```python
from build123d import *

# Parameters (mm, degrees)
SKETCH_2_R      = 2.5
EXTRUDE_1_DEPTH = 5
SKETCH_3_R      = 10
EXTRUDE_2_DEPTH = 1
EXTRUDE_3_DEPTH = 3
CHAMFER_1_SIZE  = 0.5


with BuildPart() as part:
    # 草图2 → 凸台-拉伸1 (new body)
    with BuildSketch(Plane(origin=(0, 0, 0), x_dir=(1, 0, 0), z_dir=(0, 1, 0))):
        with Locations(Location((0, 0, 0), (0, 0, 270))):
            Circle(SKETCH_2_R)
    extrude(amount=EXTRUDE_1_DEPTH)

    # 草图3 → 凸台-拉伸2 (add)
    with BuildSketch(Plane(origin=(0, 5, 0), x_dir=(1, 0, 0), z_dir=(0, 1, 0))):
        with Locations(Location((0, 0, 0), (0, 0, 270))):
            Circle(SKETCH_3_R)
    extrude(amount=EXTRUDE_2_DEPTH)

    # 草图4 → 凸台-拉伸3 (add)
    with BuildSketch(Plane(origin=(0, 6, 0), x_dir=(1, 0, 0), z_dir=(0, 1, 0))):
        Polygon((3.464101615, 6), (-3.464101615, 6), (-6.92820323, 0), (-3.464101615, -6), (3.464101615, -6), (6.92820323, 0), align=None)
    extrude(amount=EXTRUDE_3_DEPTH)

    # 草图8 → 切除-旋转1 (revolve, cut)
    with BuildSketch(Plane.XY, mode=Mode.PRIVATE) as cut_revolve_1_sk:
        Polygon((-6.92820323, 9), (-5.92820323, 9), (-6.92820323, 8.422649731), align=None)
    revolve(cut_revolve_1_sk.sketch.rotate(Axis((0, 0, 0), (0, 1, 0)), 270), axis=Axis((0, 0, 0), (0, 1, 0)), mode=Mode.SUBTRACT)

    # 倒角1
    chamfer_1_edges = [part.edges().sort_by_distance(p)[0] for p in [
        (0, 0, -2.5),
    ]]
    chamfer(chamfer_1_edges, length=CHAMFER_1_SIZE)


solid = part.part
```
CAD build for the part. Positions are in the model's coordinates, mm. A direction names the side the tool comes from. Round coordinates to 2 decimals unless told otherwise and drop trailing zeros. Write each loop counter-clockwise with the first axis right and the second up, starting at its lowest first coordinate (ties: lowest second). Pieces come first, ordered by that corner, then holes. Notation, with made-up numbers: (34, -34.5) -> (81, -34.5) arc R28 cw to (81, -16.5) -> close; hole circle Ø9 at (-28.5, -29). An arc over 180 degrees is marked (long way). Answer in a Markdown table with one row per item. Add a question column.
Item 1: Saw through at A-A, the plane x = 0. Write the cut outline in (y, z).
Item 2: Drop flat-ended pins along their axis: pin 1 Ø1 at (y, z) = (7, 4.5) entering from -X; pin 2 Ø1.5 at (x, y) = (1.5, 7.5) entering from -Z; pin 3 Ø5 at (x, z) = (-3.5, -5) entering from -Y. Give the stop position or say it passes through.
Item 3: Which spindle directions (+Z, -Z, +X, -X, +Y, -Y) get a long thin tool onto all of the face, cutting with end or side? Do faces 1 (the face through (-2.44, 2.72, -0.54)), 2 (the face through (-5.172, 7.459, -3.042)), 3 (the face through (0, 7, -6)), 4 (the face through (5.22, 7.46, -2.96)), 5 (the face through (-5.22, 7.46, 2.96)). Say none if no direction does.
Item 4: Saw through at D-D, the plane y = 3. Write the cut outline in (x, z), then the cut area to 3 significant figures.
Item 5: Saw through at B-B, the plane y = 7.5. Write the cut outline in (x, z).
Item 6: Drill centre lines: line 1 (Y direction, x = 6, z = -6.5); line 2 (Y direction, x = 5.25, z = -2); line 3 (Z direction, x = -3, y = 7). Where is each one in solid material? Low to high. Write a range as from..to.
Item 7: Saw through at C-C, the plane z = -7.25. Write the cut outline in (x, y).
Findings below:
| question | item | result |
|---|---|---|
| 1 | outline | (0, -2) -> (0.5, -2.5) -> (5, -2.5) -> (5, -10) -> (6, -10) -> (6, -6) -> (8.96, -6) -> (9, -5.93) -> (9, 5.93) -> (8.96, 6) -> (6, 6) -> (6, 10) -> (5, 10) -> (5, 2.5) -> (0.5, 2.5) -> (0, 2) -> close |
| 2 | pin 1 | stops at x = -4.62 |
| 2 | pin 2 | stops at z = -6 |
| 2 | pin 3 | stops at y = 5 |
| 3 | face 1 | -Y |
| 3 | face 2 | -Z, -X, +Y |
| 3 | face 3 | -Z, +X, -X, +Y |
| 3 | face 4 | -Z, +X, +Y |
| 3 | face 5 | +Z, -X, +Y |
| 4 | outline | circle Ø5 at (0, 0) |
| 4 | area | 19.6 mm^2 |
| 5 | outline | (-6.93, 0) -> (-3.46, -6) -> (3.46, -6) -> (6.93, 0) -> (3.46, 6) -> (-3.46, 6) -> close |
| 6 | line 1 | y = 5..6 |
| 6 | line 2 | y = 5..9 |
| 6 | line 3 | z = -6..6 |
| 7 | outline | (-6.89, 5) -> (6.89, 5) -> (6.89, 6) -> (-6.89, 6) -> close |
